Part model, mm, in its own coordinate system. Face numbers are marked on the shaded views. Coordinates: 2 decimals unless noted, no trailing zeros. Loops run counter-clockwise (first coordinate to the right, second up) from the corner with the lowest first, then second, coordinate; pieces in that order, holes last. Notation, with made-up numbers: (38, 45.25) - (61, 45.25) arc R29 cw to (61, 79.25) - close; hole circle Ø4 at (-4.75, 3.25). An arc over 180 degrees is marked (long way). Use a Markdown table: item, result. Add a question column.
1) Pull direction Z, two halves, no side cores. Call the marked faces 1, 2 and 3: +Z half, -Z half, draft (parallel to the pull), parting line (faces both ways), or undercut.
2) Band-saw the part on B-B (y = 0). Give the cut face in (x, z) (1 decimal).
3) Band-saw the part on A-A (x = 0). Give the cut face in (y, z) (1 decimal).
4) Probe probe 1 along Z at (x, y) = (0, 5.7) (3 decimals); probe 2 along Y at (x, z) = (0, -2.75) (1 decimal); probe 3 along Z at (x, y) = (5, -1.25). List the from-to ranges inside material, lowest first. Write a range as [from, to].
5) Drop flat-ended pins along their axis: P1, Ø2, axis at y = -4.5, z = -6.5, coming from the -X side; P2, Ø3, axis at y = -3, z = -1.5, coming from the +X side; P3, Ø10, axis at x = -1.5, y = -2.5, coming from the -Z side (3 decimals); P4, Ø2, axis at x = -3, z = -5, coming from the -Y side. Give the stop position or say it passes through.
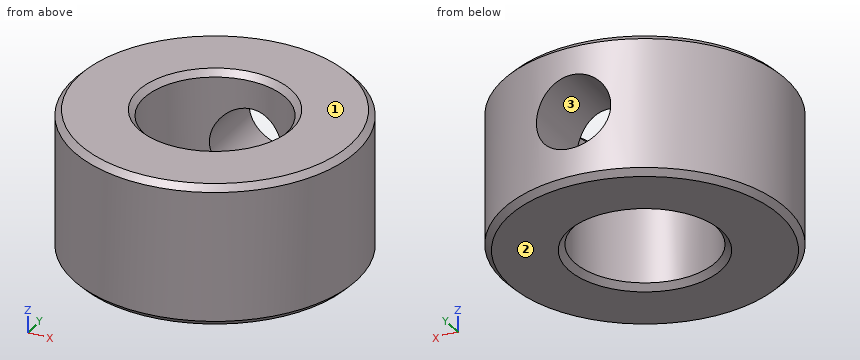
Autodesk Inventor part; units mm, degrees
ref_plane "Work Plane1" through (0, 9.525, 0) normal (0, 1, 0) x (-1, 0, 0)
ref_plane "YZ Plane" through (0, 0, 0) normal (1, 0, 0) x (0, 1, 0)
ref_plane "XY Plane" through (0, 0, 0) normal (0, 0, 1) x (1, 0, 0)
sketch "Sketch1" plane through (0, 0, 0) normal (0, 0, 1) x (1, 0, 0)
  circle A0 centre (0, 0) radius 9.525
  dimension "d0" = 19.05
extrude "Extrusion1" add sketch "Sketch1" against normal blind 9.525
sketch "Sketch2" plane through (0, 0, 0) normal (0, 0, 1) x (1, 0, 0)
  circle A0 centre (0, 0) radius 9.525
  circle A1 centre (0, 0) radius 4.7625
  dimension "d3" = 9.525
extrude "Extrusion2" cut sketch "Sketch2" against normal up to next contours A1
chamfer "Chamfer1" distance 0.3969 angle 45 4 edges at (-9.525, 0, 0) (-9.525, 0, -9.525) (-4.7625, 0, 0) (-4.7625, 0, -9.525)
ref_plane "Work Plane1" through (0, 9.525, 0) normal (0, 1, 0) x (-1, 0, 0)
sketch "Sketch3" plane through (0, 9.525, 0) normal (0, 1, 0) x (-1, 0, 0)
  line L0 (9.1281, -9.525) -> (-9.1281, -9.525)
  line L1 (9.525, -0.3969) -> (9.525, -9.1281)
  point P0 (0, 0)
  point P1 (0, -4.7625)
  point P2 (0, -9.525)
  point P3 (9.525, -4.7625)
hole "Hole1" at (0, 9.525, -4.7625) direction (0, -1, 0) diameter 4.9784 end up to surface
properties part number "Misc_ShaftCollar_Ruland_SC-6-F" material "Steel, Carbon"
Answer block:
| question | item | result |
|---|---|---|
| 1 | face 1 | +Z half |
| 1 | face 2 | -Z half |
| 1 | face 3 | undercut |
| 2 | outline | (-9.5, -9.1) - (-9.1, -9.5) - (-5.2, -9.5) - (-4.8, -9.1) - (-4.8, -0.4) - (-5.2, 0) - (-9.1, 0) - (-9.5, -0.4) - close; (4.8, -9.1) - (5.2, -9.5) - (9.1, -9.5) - (9.5, -9.1) - (9.5, -0.4) - (9.1, 0) - (5.2, 0) - (4.8, -0.4) - close |
| 3 | outline | (-9.5, -9.1) - (-9.1, -9.5) - (-5.2, -9.5) - (-4.8, -9.1) - (-4.8, -0.4) - (-5.2, 0) - (-9.1, 0) - (-9.5, -0.4) - close; (4.8, -9.1) - (5.2, -9.5) - (9.1, -9.5) - (9.5, -9.1) - (9.5, -7.3) - (4.8, -7.3) - close; (4.8, -2.3) - (9.5, -2.3) - (9.5, -0.4) - (9.1, 0) - (5.2, 0) - (4.8, -0.4) - close |
| 4 | probe 1 | [-9.525, -7.252], [-2.273, 0] |
| 4 | probe 2 | [-9.5, -4.8] |
| 4 | probe 3 | [-9.52, -0.01] |
| 5 | P1 | x = -8.86 |
| 5 | P2 | x = 9.41 |
| 5 | P3 | z = -9.525 |
| 5 | P4 | y = -9.31 |
